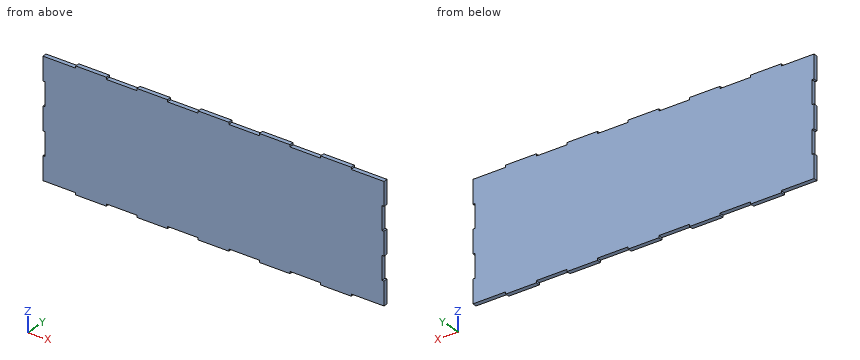
from build123d import *

# Parameters (mm, degrees)
SKETCH1_W           = 508
SKETCH1_H           = 177.8
SKETCH1_W_2         = 46.181818182
SKETCH1_H_2         = 3.175
SKETCH1_W_3         = 3.175
SKETCH1_H_3         = 35.56
BOSS_EXTRUDE1_DEPTH = 6.35


with BuildPart() as part:
    # Sketch1 → Boss-Extrude1 (new body)
    with BuildSketch(Plane(origin=(0, 0, 0), x_dir=(1, 0, 0), z_dir=(0, 1, 0))):
        with Locations((254, 88.9)):
            Rectangle(SKETCH1_W, SKETCH1_H)
        with Locations((438.727272727, 179.3875)):
            Rectangle(SKETCH1_W_2, SKETCH1_H_2)
        with Locations((346.363636364, 179.3875)):
            Rectangle(SKETCH1_W_2, SKETCH1_H_2)
        with Locations((254, 179.3875)):
            Rectangle(SKETCH1_W_2, SKETCH1_H_2)
        with Locations((161.636363636, 179.3875)):
            Rectangle(SKETCH1_W_2, SKETCH1_H_2)
        with Locations((69.272727273, 179.3875)):
            Rectangle(SKETCH1_W_2, SKETCH1_H_2)
        with Locations((-1.5875, 160.02)):
            Rectangle(SKETCH1_W_3, SKETCH1_H_3)
        with Locations((-1.5875, 88.9)):
            Rectangle(SKETCH1_W_3, SKETCH1_H_3)
        with Locations((-1.5875, 17.78)):
            Rectangle(SKETCH1_W_3, SKETCH1_H_3)
        with Locations((346.363636364, -1.5875)):
            Rectangle(SKETCH1_W_2, SKETCH1_H_2)
        with Locations((438.727272727, -1.5875)):
            Rectangle(SKETCH1_W_2, SKETCH1_H_2)
        with Locations((509.5875, 17.78)):
            Rectangle(SKETCH1_W_3, SKETCH1_H_3)
        with Locations((509.5875, 88.9)):
            Rectangle(SKETCH1_W_3, SKETCH1_H_3)
        with Locations((509.5875, 160.02)):
            Rectangle(SKETCH1_W_3, SKETCH1_H_3)
        with Locations((69.272727273, -1.5875)):
            Rectangle(SKETCH1_W_2, SKETCH1_H_2)
        with Locations((161.636363636, -1.5875)):
            Rectangle(SKETCH1_W_2, SKETCH1_H_2)
        with Locations((254, -1.5875)):
            Rectangle(SKETCH1_W_2, SKETCH1_H_2)
    extrude(amount=BOSS_EXTRUDE1_DEPTH)


solid = part.part
Source: CAD feature listing. Evaluate the final solid. Frame: model axes, mm. Give positions to 0.01 mm unless a question says otherwise; leave off trailing zeros. Loops run counter-clockwise (first coordinate to the right, second up) from the corner with the lowest first, then second, coordinate; pieces in that order, holes last. Notation, with made-up numbers: (49.5, 39) -> (99.5, 39) arc R25 ccw to (99.5, 60) -> close; hole circle Ø2 at (4.25, -18). An arc over 180 degrees is marked (long way). Use a Markdown table: item, result. Add a question column.
1) First-contact query: pin 1 (1 mm diameter, centred on x = 509, y = 3, fed in from +Z); pin 2 (1 mm diameter, centred on y = 3, z = 2, fed in from +X); pin 3 (1 mm diameter, centred on y = 4.5, z = -179, fed in from -X). Flat tips, straight axial feed; report the tip coordinate or a pass-through.
2) Line query: line 1 along Z through (x, y) = (132, 1.75); line 2 along X through (y, z) = (3.75, -117). Output: solid intervals per line, ascending. Write a range as [from, to].
3) Section query A-A, the plane x = 190.5. Return the cut outline in (y, z).
Numbers:
| question | item | result |
|---|---|---|
| 1 | pin 1 | stops at z = 0 |
| 1 | pin 2 | stops at x = 461.82 |
| 1 | pin 3 | stops at x = 46.18 |
| 2 | line 1 | z = [-177.8, 0] |
| 2 | line 2 | x = [0, 508] |
| 3 | outline | (0, -177.8) -> (6.35, -177.8) -> (6.35, 0) -> (0, 0) -> close |
